Part model, mm, in its own coordinate system. A direction names the side the tool comes from. Give positions to 0.01 mm unless a question says otherwise; leave off trailing zeros. Order: outer loops, then holes, each group sorted by start corner. A loop starts at its lowest first (then second) coordinate and runs counter-clockwise, first axis right, second up. Notation, with made-up numbers: M 28.25,2.25 L 50.25,2.25 A33 ccw 50.25,35.25 Z; hole C -5.5,-14 d5. An arc over 180 degrees is marked long. One line per question, with ' | ' between items.
```python
from build123d import *

# Parameters (mm, degrees)
BOSS_EXTRUDE1_DEPTH     = 3
SKETCH5_W               = 150
SKETCH5_H               = 20
BOSS_EXTRUDE2_DEPTH     = 3
MIRROR2_COPY_1_SKETCH_W = 150
MIRROR2_COPY_1_SKETCH_H = 20
MIRROR2_COPY_1_DEPTH    = 3
SKETCH6_W               = 23
SKETCH6_H               = 150
BOSS_EXTRUDE3_DEPTH     = 3
MIRROR4_COPY_1_SKETCH_W = 23
MIRROR4_COPY_1_SKETCH_H = 150
MIRROR4_COPY_1_DEPTH    = 3
MIRROR4_COPY_2_SKETCH_W = 23
MIRROR4_COPY_2_SKETCH_H = 150
MIRROR4_COPY_2_DEPTH    = 3
FILLET1_R               = 2


with BuildPart() as part:
    # Sketch1 → Boss-Extrude1 (new body)
    with BuildSketch(Plane.XY):
        Polygon((0, 195.984444731), (-138.581929877, 138.581929877), (-195.984444731, 0), (-138.581929877, -138.581929877), (0, -195.984444731), (138.581929877, -138.581929877), (195.984444731, 0), (138.581929877, 138.581929877), align=None)
    boss_extrude1 = extrude(amount=BOSS_EXTRUDE1_DEPTH)

    # Sketch5 → Boss-Extrude2 (add)
    with BuildSketch(Plane(origin=(-69.290964938, -167.283187304, 0), x_dir=(0.923879533, -0.382683432, 0), z_dir=(-0.382683432, -0.923879533, 0))):
        with Locations((0, -10)):
            Rectangle(SKETCH5_W, SKETCH5_H)
    boss_extrude2 = extrude(amount=-BOSS_EXTRUDE2_DEPTH)

    # Mirror1: Boss-Extrude2 across plane
    add(boss_extrude2.mirror(Plane.ZX))

    # Mirror2: Boss-Extrude2 across plane
    add(boss_extrude2.mirror(Plane(origin=(0, 0, 0), x_dir=(0, 0, 1), z_dir=(1, 0, 0))))

    # Mirror2 copy 1 sketch → Mirror2 copy 1 (add)
    with BuildSketch(Plane(origin=(69.290964938, 167.283187304, 0), x_dir=(-0.923879533, 0.382683432, 0), z_dir=(0.382683432, 0.923879533, 0))):
        with Locations((0, -10)):
            Rectangle(MIRROR2_COPY_1_SKETCH_W, MIRROR2_COPY_1_SKETCH_H)
    extrude(amount=-MIRROR2_COPY_1_DEPTH)

    # Sketch6 → Boss-Extrude3 (add)
    with BuildSketch(Plane(origin=(-167.283187304, -69.290964938, 0), x_dir=(0, 0, 1), z_dir=(-0.923879533, -0.382683432, 0))):
        with Locations((-8.5, 0)):
            Rectangle(SKETCH6_W, SKETCH6_H)
    boss_extrude3 = extrude(amount=-BOSS_EXTRUDE3_DEPTH)

    # Mirror3: Boss-Extrude3 across plane
    add(boss_extrude3.mirror(Plane.ZX))

    # Mirror4: Boss-Extrude1 across plane
    add(boss_extrude1.mirror(Plane(origin=(0, 0, 0), x_dir=(0, 0, 1), z_dir=(1, 0, 0))))

    # Mirror4 copy 1 sketch → Mirror4 copy 1 (add)
    with BuildSketch(Plane(origin=(167.283187304, 69.290964938, 0), x_dir=(0, 0, 1), z_dir=(0.923879533, 0.382683432, 0))):
        with Locations((-8.5, 0)):
            Rectangle(MIRROR4_COPY_1_SKETCH_W, MIRROR4_COPY_1_SKETCH_H)
    extrude(amount=-MIRROR4_COPY_1_DEPTH)

    # Mirror4 copy 2 sketch → Mirror4 copy 2 (add)
    with BuildSketch(Plane(origin=(167.283187304, -69.290964938, 0), x_dir=(0, 0, 1), z_dir=(0.923879533, -0.382683432, 0))):
        with Locations((-8.5, 0)):
            Rectangle(MIRROR4_COPY_2_SKETCH_W, MIRROR4_COPY_2_SKETCH_H)
    extrude(amount=-MIRROR4_COPY_2_DEPTH)

    # Fillet1
    fillet1_edges = [part.edges().sort_by_distance(p)[0] for p in [
        (-164.511548707, -68.142914641, 0),
        (-164.511548707, 68.142914641, 0),
        (164.511548707, 68.142914641, 0),
        (164.511548707, -68.142914641, 0),
        (-68.142914641, 164.511548707, 0),
        (68.142914641, 164.511548707, 0),
        (-68.142914641, -164.511548707, 0),
        (68.142914641, -164.511548707, 0),
    ]]
    fillet(fillet1_edges, radius=FILLET1_R)


solid = part.part
```
1. Probe L1, parallel to Z at x = 133, y = 95; L2, parallel to X at y = -40, z = -3.25; L3, parallel to Y at x = -166.5, z = -4.25. List the from-to ranges inside material, lowest first. Write a range as from..to.
Worked out:
L1: z = 0..3 | L2: x = -179.42..-176.17, 176.17..179.42 | L3: y = -71.18..-63.34, 63.34..71.18
2. Tool access for faces 3 (the flat face through (69.097, 164.116, -10.874)), 4 (the flat face through (-3, 3, 3)): list every direction of +Z, -Z, +X, -X, +Y, -Y with a clear straight run to the whole face (end or side of a thin tool).
Worked out:
face 3: -Z | face 4: +Z, +X, -X, +Y, -Y
3. Slice it at A-A on z = -7.25. Give the cut face in (x, y).
Worked out:
outline: M -195.98,0 L -138.58,-138.58 L 0,-195.98 L 138.58,-138.58 L 195.98,0 L 138.58,138.58 L 0,195.98 L -138.58,138.58 Z; hole M -192.74,0 L -136.29,-136.29 L 0,-192.74 L 136.29,-136.29 L 192.74,0 L 136.29,136.29 L 0,192.74 L -136.29,136.29 Z
4. Drop flat-ended pins along their axis: pin 1 (3 mm diameter, centred on y = -23.5, z = -5, fed in from -X); pin 2 (2 mm diameter, centred on x = -9, y = 102, fed in from -Z); pin 3 (12 mm diameter, centred on x = -43.5, z = -8.5, fed in from -Y). Give the stop position or say it passes through.
Worked out:
pin 1: stops at x = -186.87 | pin 2: stops at z = 0 | pin 3: stops at y = -180.45
5. Mould opens along Y. For faces 1 (the cylindrical face through (164.38, -66.97, -0.6)), 2 (the flat face through (-162, -77, -20)) say: released by +Y, released by -Y, zero draft, split by the parting line, or undercut.
Worked out:
face 1: undercut | face 2: zero draft
